Check sheet for the modelled part. Datum: model origin and axes. Units: mm. A direction names the side the tool comes from. Give positions to 0.01 mm unless a question says otherwise; leave off trailing zeros. Loops run counter-clockwise (first coordinate to the right, second up) from the corner with the lowest first, then second, coordinate; pieces in that order, holes last. Notation, with made-up numbers: (-37, 19) -> (-20, 19) arc R18 cw to (-20, 50) -> close; hole circle Ø3 at (-9.5, -32.5). An arc over 180 degrees is marked (long way). Write each question's results on one line, items separated by ' | '. Start each with the question number.
Item 1: Scan lines: line 1 along X through (y, z) = (0, 207); line 2 along X through (y, z) = (112.5, 143); line 3 along Y through (x, z) = (-196, 74.5). Record each from-to range of solid material in increasing order.
Item 2: Mould release check, pull along X, two halves, no side actions. Record for faces 3 (the face through (121, 75.749, 158)), 4 (the face through (-3, 3, 0)), 5 (the face through (-224.782, -9.893, 152.83)): pulls with the +X half, pulls with the -X half, needs draft (parallel to the pull), parting line crosses it, or undercut.
Item 3: Cross-section at B-B on x = 0. Enter the section's corners in (y, z), then the cut area to 3 significant figures.
Item 4: Cross-section at C-C on z = 87.5. Enter the section's corners in (x, y), then the cut area to 3 significant figures.
Item 5: Access from +Z, -Z, +X, -X, +Y, -Y to the whole of each face (thin tool, end or side, straight path). Record for faces 1 (the face through (16, 68, 310)), 2 (the face through (-60.907, 139.041, 157.9)).
Item 6: Cross-section at A-A on y = 0. Enter the section's corners in (x, z).
Item 7: Cross-section at D-D on x = -116. Enter the section's corners in (y, z), then the cut area to 3 significant figures.
Item 8: Gauge pin test, flat ends, axial feed: pin 1 Ø1 at (x, z) = (-123.5, 226.5) entering from -Y; pin 2 Ø3 at (x, y) = (-96, -178.5) entering from +Z; pin 3 Ø1.5 at (y, z) = (-30, 209) entering from -X. Record the tip position at first contact, or that the pin passes through.
Autodesk Inventor part; units mm, degrees
ref_plane "YZ Plane" through (0, 0, 0) normal (1, 0, 0) x (0, 1, 0)
ref_plane "XZ Plane" through (0, 0, 0) normal (0, 1, 0) x (-1, 0, 0)
ref_plane "XY Plane" through (0, 0, 0) normal (0, 0, 1) x (1, 0, 0)
sketch "Sketch1" plane through (0, 0, 0) normal (0, 0, 1) x (1, 0, 0)
  circle A0 centre (0, 0) radius 225
  dimension "d0" = 450
extrude "Extrusion1" add sketch "Sketch1" along normal blind 10
sketch "Sketch2" plane through (0, 0, 10) normal (0, 0, 1) x (1, 0, 0)
  circle A0 centre (0, 0) radius 225
  circle A1 centre (0, 0) radius 215
  dimension "d3" = 450
  dimension "d4" = 10
extrude "Extrusion2" add sketch "Sketch2" along normal blind 300
sketch "Sketch5" plane through (0, 0, 10) normal (0, 0, 1) x (1, 0, 0)
  line L0 (-80, 210.2974) -> (80, 210.2974)
  line L1 (80, 210.2974) -> (38.589, 55.7493)
  line L2 (-80, 210.2974) -> (-38.589, 55.7493)
  line L3 (-80, 210.2974) -> (80, 210.2974) construction
  line L4 (-38.589, 55.7493) -> (38.589, 55.7493)
  circle A0 centre (0, 0) radius 225
  dimension "d31" = 160
  dimension "d32" = 160
  dimension "d33" = 75
  dimension "d34" = 160
  dimension "d35" = 75
extrude "Extrusion5" add sketch "Sketch5" along normal blind 300 contours L0 L1 L4 L2
sketch "Sketch6" plane through (0, 0, 10) normal (0, 0, 1) x (1, 0, 0)
  line L0 (-77.3977, 200.5856) -> (-38.589, 55.7493)
  line L1 (-38.589, 55.7493) -> (-207.6464, 55.7493)
  arc A0 (-77.3977, 200.5856) -> (77.3977, 200.5856) centre (0, 0) ccw
  line L2 (-38.589, 55.7493) -> (38.589, 55.7493)
  line L3 (38.589, 55.7493) -> (207.6464, 55.7493)
  line L4 (43.9479, 75.7493) -> (201.2139, 75.7493)
  circle A1 centre (0, 0) radius 225
  line L5 (-43.9479, 75.7493) -> (-211.8656, 75.7493)
  line L6 (-43.9479, 75.7493) -> (-38.589, 55.7493)
  line L7 (43.9479, 75.7493) -> (38.589, 55.7493)
  arc A2 (207.6464, 55.7493) -> (201.2139, 75.7493) centre (0, 0) ccw
  arc A3 (-201.2139, 75.7493) -> (-207.6464, 55.7493) centre (0, 0) ccw
  line L8 (38.589, 55.7493) -> (77.3977, 200.5856)
  dimension "d38" = 20
extrude "Extrusion6" add sketch "Sketch6" along normal blind 300 contours L0 L1 A0 L5 | L7 L4 A0 L3
sketch "Sketch7" plane through (0, 0, 10) normal (0, 0, 1) x (1, 0, 0)
  arc A0 (-77.3977, 200.5856) -> (-201.2139, 75.7493) centre (0, 0) ccw
  line L0 (-77.3977, 200.5856) -> (-43.9479, 75.7493)
  line L1 (-43.9479, 75.7493) -> (-201.2139, 75.7493)
  line L2 (-207.6464, 55.7493) -> (207.6464, 55.7493)
  arc A1 (-207.6464, 55.7493) -> (207.6464, 55.7493) centre (0, 0) ccw
  line L3 (201.2139, 75.7493) -> (43.9479, 75.7493)
  line L4 (43.9479, 75.7493) -> (77.3977, 200.5856)
  arc A2 (201.2139, 75.7493) -> (77.3977, 200.5856) centre (0, 0) ccw
  line L5 (44.7214, 210.2974) -> (-44.7214, 210.2974)
  arc A3 (44.7214, 210.2974) -> (-44.7214, 210.2974) centre (0, 0) ccw
  circle A4 centre (0, 0) radius 225
extrude "Extrusion7" add sketch "Sketch7" along normal blind 300 contours L5 A3
properties part number "BA001" material "ABS Plastic"
Answer sheet:
1) line 1: x = -225 to -215, 215 to 225 | line 2: x = -194.86 to -183.22, -53.8 to 53.8, 183.22 to 194.86 | line 3: y = -110.49 to -88.37, 55.75 to 75.75, 88.37 to 110.49
2) face 3: undercut | face 4: needs draft | face 5: parting line crosses it
3) outline: (-225, 0) -> (225, 0) -> (225, 310) -> (55.75, 310) -> (55.75, 10) -> (-215, 10) -> (-215, 310) -> (-225, 310) -> close | area: 58,300 mm²
4) outline: circle Ø450 at (0, 0); hole (-207.65, 55.75) arc R215 ccw (long way) to (207.65, 55.75) -> close; hole (-201.21, 75.75) -> (-43.95, 75.75) -> (-77.4, 200.59) arc R215 ccw to start; hole (43.95, 75.75) -> (201.21, 75.75) arc R215 ccw to (77.4, 200.59) -> close | area: 38,700 mm²
5) face 1: +Z, +X, -X, +Y, -Y | face 2: +Z
6) outline: (-225, 0) -> (225, 0) -> (225, 310) -> (215, 310) -> (215, 10) -> (-215, 10) -> (-215, 310) -> (-225, 310) -> close
7) outline: (-192.79, 0) -> (192.79, 0) -> (192.79, 310) -> (181.02, 310) -> (181.02, 10) -> (75.75, 10) -> (75.75, 310) -> (55.75, 310) -> (55.75, 10) -> (-181.02, 10) -> (-181.02, 310) -> (-192.79, 310) -> close | area: 16,900 mm²
8) pin 1: stops at y = -188.4 | pin 2: stops at z = 10 | pin 3: stops at x = -223.09
